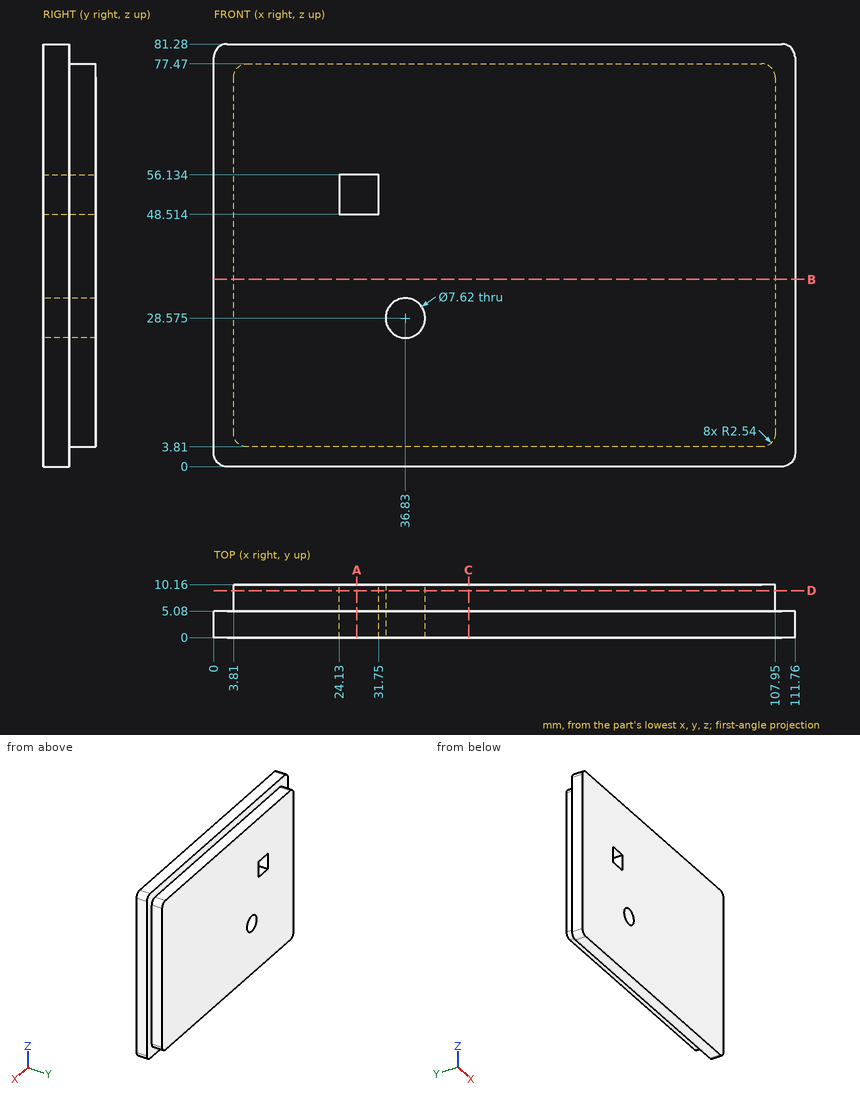
Part print with two shaded views. Sizes in mm from the minimum x, y, z corner. Round coordinates to 2 decimals unless told otherwise and drop trailing zeros. Order: outer loops, then holes, each group sorted by start corner. A loop starts at its lowest first (then second) coordinate and runs counter-clockwise, first axis right, second up.
(1) Pin check, flat tips, straight feed: pin 1 (1.5 mm diameter, centred on x = 84, z = 16, fed in from -Y); pin 2 (4 mm diameter, centred on y = 8, z = 34.5, fed in from +X); pin 3 (1.5 mm diameter, centred on y = 7, z = 40, fed in from -X); pin 4 (4 mm diameter, centred on x = 46, y = 8.5, fed in from +Z). Stop position of each tip, or through.
(2) Band-saw the part on C-C (x = 49). List the corners of the cut face in (y, z).
(3) Band-saw the part on B-B (z = 36). List the corners of the cut face in (x, y), then the cut area to 3 significant figures.
(4) Band-saw the part on A-A (x = 27.5). List the corners of the cut face in (y, z).
(5) Band-saw the part on D-D (y = 9). List the corners of the cut face in (x, z) (3 decimals), then the cut area to 3 significant figures.
(6) Drill centre lines: line 1 (X direction, y = 9.75, z = 51); line 2 (X direction, y = 2.5, z = 49.5); line 3 (Z direction, x = 36.83, y = 5.5) (3 decimals). Where is each one in solid material? Low to high.
Verdict:
1. pin 1: stops at y = 0
1. pin 2: stops at x = 107.95
1. pin 3: stops at x = 3.81
1. pin 4: stops at z = 77.47
2. outline: (0, 0) - (5.08, 0) - (5.08, 3.81) - (10.16, 3.81) - (10.16, 77.47) - (5.08, 77.47) - (5.08, 81.28) - (0, 81.28) - close
3. outline: (0, 0) - (111.76, 0) - (111.76, 5.08) - (107.95, 5.08) - (107.95, 10.16) - (3.81, 10.16) - (3.81, 5.08) - (0, 5.08) - close
3. area: 1,100 mm2
4. outline: (0, 0) - (5.08, 0) - (5.08, 3.81) - (10.16, 3.81) - (10.16, 48.51) - (0, 48.51) - close; (0, 56.13) - (10.16, 56.13) - (10.16, 77.47) - (5.08, 77.47) - (5.08, 81.28) - (0, 81.28) - close
5. outline: (3.81, 6.35) arc R2.54 ccw to (6.35, 3.81) - (105.41, 3.81) arc R2.54 ccw to (107.95, 6.35) - (107.95, 74.93) arc R2.54 ccw to (105.41, 77.47) - (6.35, 77.47) arc R2.54 ccw to (3.81, 74.93) - close; hole (24.13, 48.514) - (31.75, 48.514) - (31.75, 56.134) - (24.13, 56.134) - close; hole circle Ø7.62 at (36.83, 28.575)
5. area: 7,560 mm2
6. line 1: x = 3.81 to 24.13, 31.75 to 107.95
6. line 2: x = 0 to 24.13, 31.75 to 111.76
6. line 3: z = 3.81 to 24.765, 32.385 to 77.47
